For this review, use the dimensioned drawing (mm, ordinates from the lowest corner) and the shaded views. A direction names the side the tool comes from. Round coordinates to 2 decimals unless told otherwise and drop trailing zeros. Write each loop counter-clockwise with the first axis right and the second up, starting at its lowest first coordinate (ties: lowest second). Pieces come first, ordered by that corner, then holes. Notation, with made-up numbers: M 17,87 L 34,87 A17 ccw 34,117 Z; hole C 62.5,47 d2. An arc over 180 degrees is marked long. Use CSV: the item, a comma, the result in double quotes.
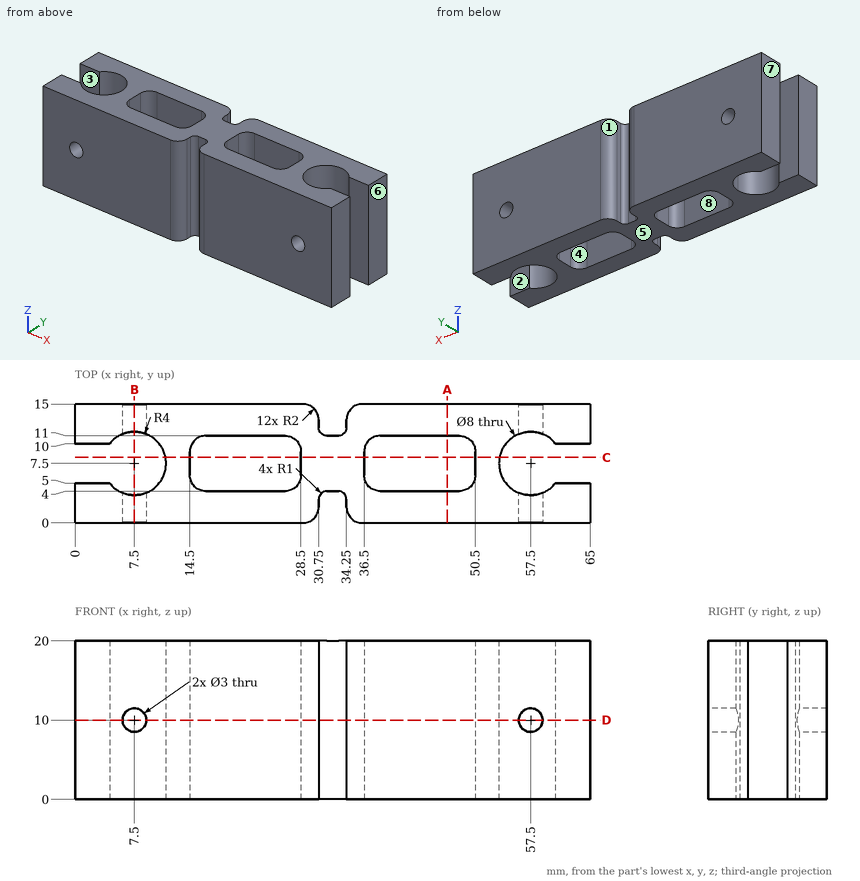
1) Add section C-C on y = 8.25. Write out the cut boundary in (x, z).
Answers:
outline,"M 11.43,0 L 14.5,0 L 14.5,20 L 11.43,20 Z; M 28.5,0 L 36.5,0 L 36.5,20 L 28.5,20 Z; M 50.5,0 L 53.57,0 L 53.57,20 L 50.5,20 Z"
2) Add section D-D on z = 10. Give the number of separate pieces and of enclosed holes in the cut face, then the cut area to 3 significant figures.
Answers:
separate pieces,"5"
enclosed holes,"2"
area,"574 mm²"
3) Machinability: for the marked faces 1, 2, 3 and 4, which of the approach directions +Z, -Z, +X, -X, +Y, -Y give a long, thin tool a straight path to every point of the face, cutting with its end or side? Answer none if there is none.
Answers:
face 1,"+Z, -Z, +Y"
face 2,"+Z, -Z, +X"
face 3,"+Z, -Z, -X"
face 4,"+Z, -Z"
4) The part is to be moulded in two halves that separate along X. For the marked faces 5, 6, 7 and 8, say which applies: released by +X, released by -X, zero draft, split by the parting line, or undercut.
Answers:
face 5,"zero draft"
face 6,"released by +X"
face 7,"released by -X"
face 8,"undercut"
5) Wall thickness on line 1 along Y through (x, z) = (47.5, 6); line 2 along Y through (x, z) = (57.5, 16.25); line 3 along Z through (x, y) = (57.5, 13.5): over which ranges is each line inside the solid? List them lowest first. Write a range as [from, to].
Answers:
line 1,"[0, 4], [11, 15]"
line 2,"[0, 3.5], [11.5, 15]"
line 3,"[0, 8.5], [11.5, 20]"
6) For pin 1 Ø3.5 at (x, z) = (57.5, 10) entering from -Y; pin 2 Ø2.5 at (x, z) = (7.5, 10) entering from +Y; pin 3 Ø3.5 at (y, z) = (7, 13) entering from -X; pin 4 Ø3.5 at (y, z) = (7.5, 6.5) entering from +X, all flat-tipped, find the tip position at first contact; note any pin that passes through.
Answers:
pin 1,"y = 0"
pin 2,"through"
pin 3,"x = 10.81"
pin 4,"x = 53.9"
7) Add section B-B on x = 7.5. Write out the cut boundary in (y, z).
Answers:
outline,"M 0,0 L 3.5,0 L 3.5,8.5 L 0,8.5 Z; M 0,11.5 L 3.5,11.5 L 3.5,20 L 0,20 Z; M 11.5,0 L 15,0 L 15,8.5 L 11.5,8.5 Z; M 11.5,11.5 L 15,11.5 L 15,20 L 11.5,20 Z"
8) Add section A-A on x = 47. Write out the cut boundary in (y, z).
Answers:
outline,"M 0,0 L 4,0 L 4,20 L 0,20 Z; M 11,0 L 15,0 L 15,20 L 11,20 Z"
